Geometry: see drawing. Coordinates: mm, zero at the bounding-box minimum. A direction names the side the tool comes from. Coordinates: 2 decimals unless noted, no trailing zeros. Write each loop counter-clockwise with the first axis right and the second up, starting at its lowest first coordinate (ties: lowest second). Pieces come first, ordered by that corner, then holes. Notation, with made-up numbers: (-30.75, -30.5) - (1.25, -30.5) arc R28 cw to (1.25, 3.5) - close; hole circle Ø9 at (77, 76). An arc over 180 degrees is marked (long way). Use a Markdown table: item, result. Add a question column.
Q1. Material intervals for probe 1 along Y at (x, z) = (7, 8.5); probe 2 along Y at (x, z) = (21, 0.7); probe 3 along Y at (x, z) = (6, 8), sorted ascending. Write a range as from..to.
Q2. Section query A-A (x = 21). Return the cut outline in (y, z).
Q3. Section query D-D (y = 3). Return the cut outline in (x, z).
Q4. Section query C-C (z = 6.5). Return the cut outline in (x, y), then the cut area to 3 significant figures.
Q5. Mould query, pull axis Y, two halves, no side actions, for the marked faces 1, 2, 3 and 4. Classes: released by +Y, released by -Y, zero draft, split by the parting line, or undercut.
Q6. Set-up query: the marked faces 5 and 6. Return all of +Z, -Z, +X, -X, +Y, -Y with unobstructed straight access to the full face (end or side cutting, diameter ignored); none if empty.
Q7. Pin query (flat end, axial travel): P1, Ø15, axis at x = 21, y = 21, coming from the +Z side; P2, Ø8, axis at x = 16.5, y = 26.5, coming from the +Z side; P3, Ø1, axis at y = 29, z = 4, coming from the -X side; P4, Ø5, axis at y = 31.5, z = 2, coming from the +X side. Return the tip coordinate at first contact, or that it passes through.
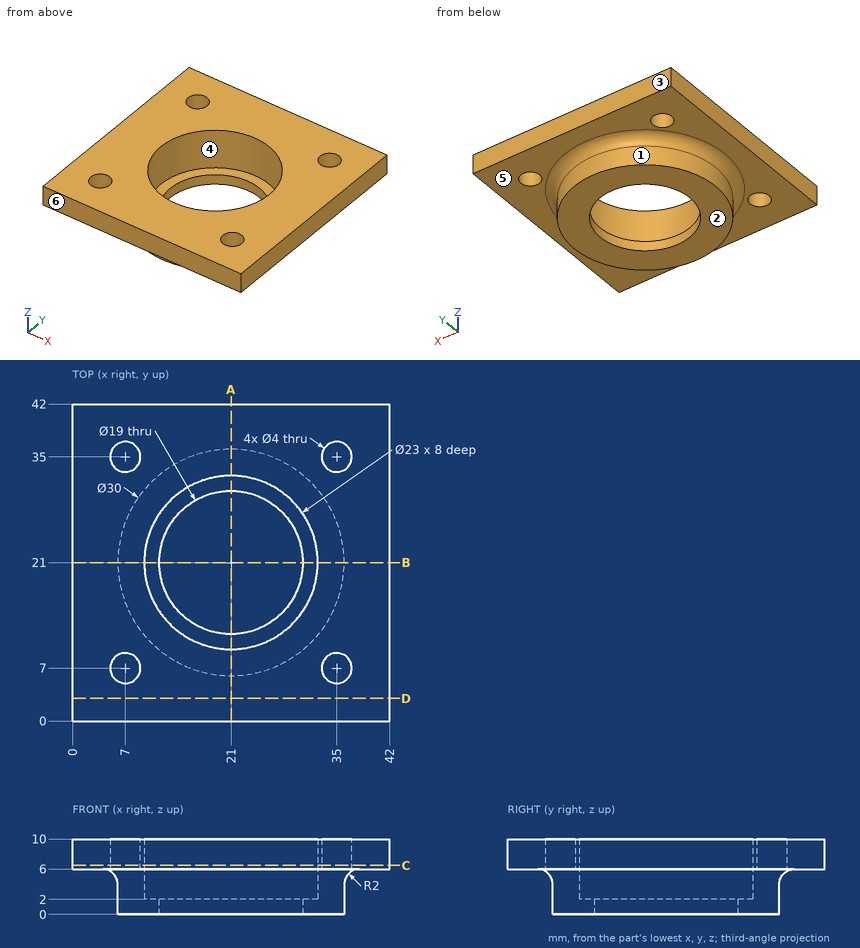
Values follow:
| question | item | result |
|---|---|---|
| 1 | probe 1 | 0..5, 9..33, 37..42 |
| 1 | probe 2 | 6..11.5, 30.5..36 |
| 1 | probe 3 | 0..5.27, 8.73..33.27, 36.73..42 |
| 2 | outline | (0, 6) - (4, 6) arc R2 cw to (6, 4) - (6, 0) - (11.5, 0) - (11.5, 2) - (9.5, 2) - (9.5, 10) - (0, 10) - close; (30.5, 0) - (36, 0) - (36, 4) arc R2 cw to (38, 6) - (42, 6) - (42, 10) - (32.5, 10) - (32.5, 2) - (30.5, 2) - close |
| 3 | outline | (0, 6) - (42, 6) - (42, 10) - (0, 10) - close |
| 4 | outline | (0, 0) - (42, 0) - (42, 42) - (0, 42) - close; hole circle Ø4 at (7, 7); hole circle Ø4 at (7, 35); hole circle Ø23 at (21, 21); hole circle Ø4 at (35, 7); hole circle Ø4 at (35, 35) |
| 4 | area | 1,300 mm2 |
| 5 | face 1 | split by the parting line |
| 5 | face 2 | zero draft |
| 5 | face 3 | released by +Y |
| 5 | face 4 | undercut |
| 6 | face 5 | -Z |
| 6 | face 6 | +Z, -Z, +X, -X, -Y |
| 7 | P1 | through |
| 7 | P2 | z = 2 |
| 7 | P3 | x = 8.01 |
| 7 | P4 | x = 33.69 |
